For this review, take the finished solid that the model builds, in its own axes (mm). A direction names the side the tool comes from. Give positions to 0.01 mm unless a question says otherwise; leave off trailing zeros. Write each loop counter-clockwise with the first axis right and the second up, starting at its lowest first coordinate (ties: lowest second). Pieces come first, ordered by that corner, then holes. Notation, with made-up numbers: (84.5, 62) -> (107.5, 62) arc R25 ccw to (107.5, 91) -> close; hole circle Ø11 at (9, 22). An arc over 180 degrees is marked (long way). Answer as CSV lines item,"result".
```python
from build123d import *

# Parameters (mm, degrees)
SKETCH3_W           = 152.4
SKETCH3_H           = 152.4
BOSS_EXTRUDE1_DEPTH = 3.175
SKETCH4_R           = 1.8
SKETCH4_W           = 47.1
SKETCH4_H           = 27.5
CUT_EXTRUDE1_DEPTH  = 10
SKETCH5_R           = 3.175
CUT_EXTRUDE2_DEPTH  = 5


with BuildPart() as part:
    # Sketch3 → Boss-Extrude1 (new, symmetric)
    with BuildSketch(Plane(origin=(0, 0, 0), x_dir=(1, 0, 0), z_dir=(0, 1, 0))):
        Rectangle(SKETCH3_W, SKETCH3_H)
    extrude(amount=BOSS_EXTRUDE1_DEPTH, both=True)

    # Sketch4 → Cut-Extrude1 (cut)
    with BuildSketch(Plane(origin=(0, 3.175, 0), x_dir=(1, 0, 0), z_dir=(0, 1, 0))):
        with Locations(Location((0, 60.361146992, 0), (0, 0, 270))):
            Circle(SKETCH4_R)
        with Locations(Location((0, 20.361146992, 0), (0, 0, 90))):
            Circle(SKETCH4_R)
        with Locations((0, 40.361146992)):
            Rectangle(SKETCH4_W, SKETCH4_H)
    extrude(amount=-CUT_EXTRUDE1_DEPTH, mode=Mode.SUBTRACT)

    # Sketch5 → Cut-Extrude2 (cut, symmetric)
    with BuildSketch(Plane(origin=(0, 0, 0), x_dir=(1, 0, 0), z_dir=(0, 1, 0))):
        with Locations(Location((-53.096867931, -55.98098713, 0), (0, 0, 90))):
            Circle(SKETCH5_R)
        with Locations(Location((53.096867931, -55.98098713, 0), (0, 0, 90))):
            Circle(SKETCH5_R)
    extrude(amount=CUT_EXTRUDE2_DEPTH, both=True, mode=Mode.SUBTRACT)


solid = part.part
```
Q1. Add section C-C (y = -1). Write out the cut boundary in (x, z) (3 decimals), plus the area to 3 significant figures.
Answer block:
outline,"(-76.2, -76.2) -> (76.2, -76.2) -> (76.2, 76.2) -> (-76.2, 76.2) -> close; hole circle Ø6.35 at (-53.097, 55.981); hole (-23.55, -54.111) -> (23.55, -54.111) -> (23.55, -26.611) -> (-23.55, -26.611) -> close; hole circle Ø3.6 at (0, -60.361); hole circle Ø3.6 at (0, -20.361); hole circle Ø6.35 at (53.097, 55.981)"
area,"21,800 mm2"
Q2. Clearance check with flat-ended pins moving along their axes: pin 1 (3 mm diameter, centred on x = 0, z = -60.36, fed in from +Y); pin 2 (7.5 mm diameter, centred on x = -53.1, z = 55.98, fed in from -Y) (3 decimals). State where each tip first meets the part, or that it passes through.
Answer block:
pin 1,"passes through"
pin 2,"stops at y = -3.175"
Q3. To check wall thickness, follow probe 1 along X at (y, z) = (-2.25, 58); probe 2 along Z at (x, y) = (14, 2); probe 3 along X at (y, z) = (1, -19). State the ranges of each line that lie inside material, in increasing order. Write a range as [from, to].
Answer block:
probe 1,"x = [-76.2, -55.55], [-50.65, 50.65], [55.55, 76.2]"
probe 2,"z = [-76.2, -54.11], [-26.61, 76.2]"
probe 3,"x = [-76.2, -1.18], [1.18, 76.2]"
Q4. For faces 1 (the flat face through (-23.55, 0, -40)), 2 (the flat face through (-1, 3.175, -1)), list the 3-axis set-ups (+Z, -Z, +X, -X, +Y, -Y) from which the entire face can be reached by the end or side of a thin tool; tool diameter is ignored.
Answer block:
face 1,"+Y, -Y"
face 2,"+Z, -Z, +X, -X, +Y"
Q5. Add section B-B (x = 0). Write out the cut boundary in (y, z) (3 decimals).
Answer block:
outline,"(-3.175, -76.2) -> (3.175, -76.2) -> (3.175, -62.161) -> (-3.175, -62.161) -> close; (-3.175, -58.561) -> (3.175, -58.561) -> (3.175, -54.111) -> (-3.175, -54.111) -> close; (-3.175, -26.611) -> (3.175, -26.611) -> (3.175, -22.161) -> (-3.175, -22.161) -> close; (-3.175, -18.561) -> (3.175, -18.561) -> (3.175, 76.2) -> (-3.175, 76.2) -> close"
Q6. Add section A-A (z = -39). Write out the cut boundary in (x, y) (3 decimals), plus the area to 3 significant figures.
Answer block:
outline,"(-76.2, -3.175) -> (-23.55, -3.175) -> (-23.55, 3.175) -> (-76.2, 3.175) -> close; (23.55, -3.175) -> (76.2, -3.175) -> (76.2, 3.175) -> (23.55, 3.175) -> close"
area,"669 mm2"
Q7. Draft analysis for pull direction Z (two halves, no side actions). For faces 3 (the flat face through (-76.2, 0, 1)), 4 (the flat face through (0, 0, -54.111)), 5 (the cylindrical face through (-0.079, 0.044, -18.563)), 6 (the flat face through (-1, 0, -76.2)), state which applies: released by +Z, released by -Z, zero draft, split by the parting line, or undercut.
Answer block:
face 3,"zero draft"
face 4,"undercut"
face 5,"undercut"
face 6,"released by -Z"
